Design review of the part built by this model. Coordinates are the model's own, in mm. Coordinates: 2 decimals unless noted, no trailing zeros. Write each loop counter-clockwise with the first axis right and the second up, starting at its lowest first coordinate (ties: lowest second). Pieces come first, ordered by that corner, then holes. Notation, with made-up numbers: (85.5, -20.5) - (126.5, -20.5) arc R28 cw to (126.5, 15.5) - close; hole circle Ø8 at (40, 44). An arc over 180 degrees is marked (long way). Answer as a JSON object with one key per item and string values.
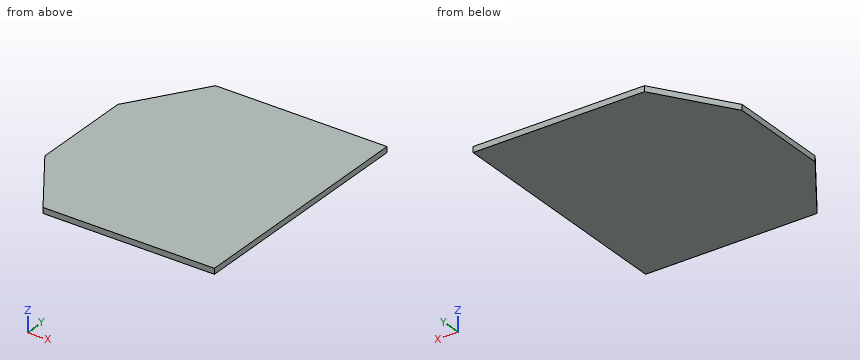
Autodesk Fusion 360 part; units mm, degrees
sketch "Sketch1" plane through (0, 0, 0) normal (0, 0, 1) x (1, 0, 0)
  line L0 (6.47, -5.82) -> (-6.47, -5.82)
  line L1 (-6.47, -5.82) -> (-6.47, 5.82)
  line L2 (-6.47, 5.82) -> (6.47, 5.82)
  line L3 (6.47, 5.82) -> (6.47, -5.82)
  line L4 (6.47, -5.82) -> (-6.47, 5.82) construction
  line L5 (-6.47, -5.82) -> (6.47, 5.82) construction
  line L6 (6.47, -5.82) -> (-6.47, -5.82)
  line L7 (-6.47, -5.82) -> (-6.47, 3.338)
  line L8 (-6.47, 3.338) -> (6.47, 3.338)
  line L9 (6.47, 3.338) -> (6.47, -5.82)
  line L10 (6.47, 3.338) -> (-6.47, 3.338)
  line L11 (-6.47, 3.338) -> (-6.47, -2.13)
  line L12 (-6.47, -2.13) -> (6.47, -2.13)
  line L13 (6.47, -2.13) -> (6.47, 3.338)
  line L14 (6.47, -5.82) -> (-2.649, -5.82)
  line L15 (-2.649, -5.82) -> (-2.649, 5.82)
  line L16 (-2.649, 5.82) -> (6.47, 5.82)
  line L17 (6.47, 5.82) -> (6.47, -5.82)
  line L18 (-2.649, -5.82) -> (-5.17, -5.82)
  line L19 (-5.17, -5.82) -> (-5.17, -2.13)
  line L20 (-5.17, -2.13) -> (-2.649, -2.13)
  line L21 (-2.649, -2.13) -> (-2.649, -5.82)
  line L22 (-2.649, 3.338) -> (-5.17, 3.338)
  line L23 (-5.17, 3.338) -> (-5.17, 5.82)
  line L24 (-5.17, 5.82) -> (-2.649, 5.82)
  line L25 (-2.649, 5.82) -> (-2.649, 3.338)
  line L26 (6.47, -5.82) -> (-5.17, -5.82)
  line L27 (-5.17, -5.82) -> (-5.17, 7.12)
  line L28 (-5.17, 7.12) -> (6.47, 7.12)
  line L29 (6.47, 7.12) -> (6.47, -5.82)
  line L30 (-2.649, 5.82) -> (-2.649, 7.12)
  line L31 (-2.649, 7.12) -> (-5.17, 3.338)
  line L32 (-5.17, -2.13) -> (-2.649, -5.82)
  dimension "d1" = 12.94
  dimension "d2" = 11.64
  dimension "d3" = 9.158
  dimension "d4" = 5.468
  dimension "d5" = 9.119
  dimension "d6" = 2.521
  dimension "d7" = 2.521
  dimension "d8" = 12.94
extrude "Extrude1" add sketch "Sketch1" along normal blind 0.1 contours L0 L3 L6 L9 L12 L14 L15 L17 L21 L26 L29 | L12 L15 L20 L21 L32 | L3 L8 L9 L10 L12 L13 L15 L17 L29 | L8 L10 L12 L15 L20 L22 L27 | L2 L3 L8 L10 L15 L16 L17 L25 L29 | L2 L8 L10 L15 L22 L24 L25 L31 | L2 L16 L28 L29 L30 | L2 L24 L30 L31
extrude "Extrude2" add 1 faces at (2.59, 1.546, 0.1) along direction (0, 0, 1) blind 0.2
(1) Take a section at C-C, the plane y = -4.75. Write out the cut boundary in (x, z).
Solved:
{"outline": "(-3.38, 0) - (6.47, 0) - (6.47, 0.3) - (-3.38, 0.3) - close"}
(2) Take a section at A-A, the plane z = 0.25. Write out the cut boundary in (x, y), and give its area (3 significant figures).
Solved:
{"outline": "(-5.17, -2.13) - (-2.65, -5.82) - (6.47, -5.82) - (6.47, 7.12) - (-2.65, 7.12) - (-5.17, 3.34) - close", "area": "141 mm^2"}
(3) To check wall thickness, follow line 1 (X direction, y = 3.75, z = 0.05); line 2 (Y direction, x = -4, z = 0.2); line 3 (X direction, y = 5, z = 0.25). State the ranges of each line that lie inside material, in increasing order. Write a range as from..to.
Solved:
{"line 1": "x = -4.9..6.47", "line 2": "y = -3.84..5.09", "line 3": "x = -4.06..6.47"}
(4) Take a section at B-B, the plane x = -3.25. Write out the cut boundary in (y, z), and give its area (3 significant figures).
Solved:
{"outline": "(-4.94, 0) - (6.22, 0) - (6.22, 0.3) - (-4.94, 0.3) - close", "area": "3.35 mm^2"}
